Here's how the part is built. I have some questions about the finished solid (model axes, mm). A direction names the side the tool comes from. Coordinates: 2 decimals unless noted, no trailing zeros. Write each loop counter-clockwise with the first axis right and the second up, starting at its lowest first coordinate (ties: lowest second). Pieces come first, ordered by that corner, then holes.
```python
from build123d import *

# Parameters (mm, degrees)
F0_R     = 4.25
F1_DEPTH = 5
F2_R     = 2.5
F3_DEPTH = 15
F5_DEPTH = 3.2
F6_R     = 0.5


with BuildPart() as f1:
    # F0 (on Top) → F1 (new body)
    with BuildSketch(Plane.XY):
        Circle(F0_R)
    extrude(amount=F1_DEPTH)

    # F2 (on face) → F3 (join)
    with BuildSketch(Plane(origin=(0, 0, 0), x_dir=(1, 0, 0), z_dir=(0, 0, -1))):
        Circle(F2_R)
    extrude(amount=F3_DEPTH)

    # F4 (on face) → F5 (cut)
    with BuildSketch(Plane.XY.offset(5)):
        Polygon((-1.154701, -2), (1.154701, -2), (2.309401, 0), (1.154701, 2), (-1.154701, 2), (-2.309401, 0), align=None)
    extrude(amount=-F5_DEPTH, mode=Mode.SUBTRACT)

    # F6
    f6_edges = [f1.edges().sort_by_distance(p)[0] for p in [
        (-4.25, 0, 5),
        (-4.25, 0, 0),
    ]]
    fillet(f6_edges, radius=F6_R)


solid = f1.part
```
1) Imagine slicing it at B-B on z = -7. Please give me the cut outline in (x, y).
Values follow:
outline: circle Ø5 at (0, 0)
2) Imagine slicing it at A-A on x = 0. Please give me the cut outline in (y, z).
Values follow:
outline: (-4.25, 0.5) arc R0.5 ccw to (-3.75, 0) - (-2.5, 0) - (-2.5, -15) - (2.5, -15) - (2.5, 0) - (3.75, 0) arc R0.5 ccw to (4.25, 0.5) - (4.25, 4.5) arc R0.5 ccw to (3.75, 5) - (2, 5) - (2, 1.8) - (-2, 1.8) - (-2, 5) - (-3.75, 5) arc R0.5 ccw to (-4.25, 4.5) - close
3) We'd pull the mould along X, two halves only. Please class faces 1 (the face through (0, 0, -15)), 2 (the face through (0, 0, 1.8)), 3 (the face through (2.285, 3.584, 2.472)): pulls with the +X half, pulls with the -X half, needs draft (parallel to the pull), parting line crosses it, or undercut.
Values follow:
face 1: needs draft
face 2: undercut
face 3: parting line crosses it
4) Will these pins go through, and if not, where does the flat tip stop? pin 1 (1.8 mm diameter, centred on x = -0.5, z = 3.5, fed in from +Y); pin 2 (1 mm diameter, centred on y = 2.5, z = -12.5, fed in from +X); pin 3 (2 mm diameter, centred on x = 0.5, y = -0.5, fed in from +Z); pin 4 (4 mm diameter, centred on x = 2, z = -8, fed in from +Y).
Values follow:
pin 1: stops at y = 4.25
pin 2: stops at x = 1.5
pin 3: stops at z = 1.8
pin 4: stops at y = 2.5
5) On a 3-axis mill with a long thin cutter (end or side, diameter ignored), from which of +Z, -Z, +X, -X, +Y, -Y can I reach the whole of each face in a straight line? I mean faces 4 (the face through (0, 3, 0)), 5 (the face through (2, -2, 5)), 6 (the face through (0, 2, 3)). Say none if no direction works.
Values follow:
face 4: -Z
face 5: +Z, +X, -X, +Y, -Y
face 6: +Z
6) I need wall thicknesses on probe 1 along X at (y, z) = (1.5, -11); probe 2 along Y at (x, z) = (2.25, 3.25); probe 3 along Z at (x, y) = (2.25, -1.5). Which ranges of each line are inside material? Lowest first, please.
Values follow:
probe 1: x = -2 to 2
probe 2: y = -3.61 to -0.1, 0.1 to 3.61
probe 3: z = 0 to 5
